```python
from build123d import *

# Parameters (mm, degrees)
EXTRUDE_1_DEPTH     = 30
SKETCH_2_R          = 5
CUT_EXTRUDE_1_DEPTH = 30
M5X0_5_1_D          = 4.5
M5X0_5_1_DEPTH      = 10
M5X0_5_1_TIP        = 1.351936393
SKETCH_7_W          = 17
SKETCH_7_H          = 0.5
CUT_EXTRUDE_2_DEPTH = 41.496913463
CHAMFER_1_SIZE      = 1
FILLET_1_R          = 1


with BuildPart() as part:
    # 草图1 → 凸台-拉伸1 (new body)
    with BuildSketch(Plane(origin=(0, 0, 0), x_dir=(1, 0, 0), z_dir=(0, 1, 0))):
        Polygon((-22, 0), (22, 0), (22, -15), (5, -15), (5, -16), (-5, -16), (-5, -15), (-22, -15), align=None)
    extrude(amount=EXTRUDE_1_DEPTH)

    # 草图2 → 切除-拉伸1 (cut)
    with BuildSketch(Plane.XZ):
        with Locations(Location((0, 7.6, 0), (0, 0, 270))):
            Circle(SKETCH_2_R)
    extrude(amount=-CUT_EXTRUDE_1_DEPTH, mode=Mode.SUBTRACT)

    # M5X0.5 螺纹孔的螺纹孔钻头1
    with Locations(Plane(origin=(0, 0, 0), x_dir=(-1, 0, 0), z_dir=(0, 0, -1))):
        with Locations((-16, 24), (16, 24), (16, 6), (-16, 6)):
            Hole(M5X0_5_1_D / 2, depth=M5X0_5_1_DEPTH)
            with Locations((0, 0, -(M5X0_5_1_DEPTH + M5X0_5_1_TIP / 2))):  # 118° drill point
                Cone(0, M5X0_5_1_D / 2, M5X0_5_1_TIP, mode=Mode.SUBTRACT)

    # 草图7 → 切除-拉伸2 (cut, through all)
    with BuildSketch(Plane.XZ):
        with Locations((0, 0.25)):
            Rectangle(SKETCH_7_W, SKETCH_7_H)
    extrude(amount=-CUT_EXTRUDE_2_DEPTH, mode=Mode.SUBTRACT)

    # 倒角1
    chamfer_1_edges = [part.edges().sort_by_distance(p)[0] for p in [
        (-5, 15, 15),
        (5, 15, 15),
        (0, 30, 12.6),
        (0, 0, 12.6),
    ]]
    chamfer(chamfer_1_edges, length=CHAMFER_1_SIZE - 0.0001)  # a hair under: the kernel refuses the full size

    # 圆角1
    fillet_1_edges = [part.edges().sort_by_distance(p)[0] for p in [
        (-22, 15, 15),
        (-22, 15, 0),
        (22, 15, 0),
        (22, 15, 15),
    ]]
    fillet(fillet_1_edges, radius=FILLET_1_R)


solid = part.part
```
Could you check a few things on this model? Use its own coordinates, in mm. A direction names the side the tool comes from. Round coordinates to 2 decimals unless told otherwise and drop trailing zeros. Loops run counter-clockwise (first coordinate to the right, second up) from the corner with the lowest first, then second, coordinate; pieces in that order, holes last.
Q1. I want a section at C-C (x = 0). Write out the boundary of the cut face in (y, z), and give its area (3 significant figures).
Q2. I want a section at A-A (z = 7.6). Write out the boundary of the cut face in (x, y), and give its area (3 significant figures).
Q3. Please list where these lines run through material, in increasing order: L1, parallel to Y at x = 16, z = 4.25; L2, parallel to X at y = 24, z = 2.5; L3, parallel to X at y = 6, z = 6.75.
Q4. I want a section at D-D (x = 13). Write out the boundary of the cut face in (y, z), and give its area (3 significant figures).
Q5. On a 3-axis mill with a long thin cutter (end or side, diameter ignored), from which of +Z, -Z, +X, -X, +Y, -Y can I reach the whole of each face in a straight line? I mean faces 1 (the cylindrical face through (17.038, 22.004, 5.07)), 2 (the flat face through (5.2, 30, 11.4)), 3 (the flat face through (14, 15, 15)). Say none if no direction works.
Q6. For P1, Ø2.5, axis at x = -16, y = 24, coming from the -Z side; P2, Ø4.5, axis at x = 12, y = 16.5, coming from the +Z side; P3, Ø1, axis at x = -6, y = 10, coming from the +Z side, each with a flat end and sliding along its axis, tell me the tip position at first contact or that it passes through.
Q7. Thinking about a two-plate mould opening in Z: for faces 4 (the flat face through (5.2, 0, 11.4)), 5 (the cylindrical face through (-3, 14.8, 11.6)), 6 (the conical face through (16.29, 24.26, 11.12)), 7 (the flat face through (5.5, 14.8, 15.5)), which applies, pulls with the +Z half, pulls with the -Z half, needs draft (parallel to the pull), parting line crosses it, or undercut?
Answer below:
1. outline: (0, 0.5) - (30, 0.5) - (30, 1.6) - (29, 2.6) - (1, 2.6) - (0, 1.6) - close; (0, 13.6) - (1, 12.6) - (29, 12.6) - (30, 13.6) - (30, 16) - (0, 16) - close
1. area: 163 mm2
2. outline: (-22, 0) - (-6, 0) - (-5, 1) - (-5, 29) - (-6, 30) - (-22, 30) - close; (5, 1) - (6, 0) - (22, 0) - (22, 30) - (6, 30) - (5, 29) - close; hole circle Ø4.5 at (-16, 6); hole circle Ø4.5 at (-16, 24); hole circle Ø4.5 at (16, 6); hole circle Ø4.5 at (16, 24)
2. area: 954 mm2
3. L1: y = 0 to 3.75, 8.25 to 21.75, 26.25 to 30
3. L2: x = -22 to -18.25, -13.75 to 13.75, 18.25 to 22
3. L3: x = -22 to -18.25, -13.75 to -4.93, 4.93 to 13.75, 18.25 to 22
4. outline: (0, 0) - (30, 0) - (30, 15) - (0, 15) - close
4. area: 450 mm2
5. face 1: -Z
5. face 2: +Z, -Z, +X, -X, +Y
5. face 3: +Z, +X, +Y, -Y
6. P1: stops at z = 10.6
6. P2: stops at z = 15
6. P3: stops at z = 15.5
7. face 4: needs draft
7. face 5: undercut
7. face 6: pulls with the -Z half
7. face 7: pulls with the +Z half
